```python
from build123d import *

# Parameters (mm, degrees)
F0_W      = 70
F0_H      = 52
F1_DEPTH  = 2.5
F2_R      = 0.5
F3_DEPTH  = 2
F5_DEPTH  = 7
F6_W      = 44
F6_H      = 52
F7_DEPTH  = 25
F10_W     = 48
F10_H     = 52
F11_DEPTH = 1.25
F12_W     = 48
F12_H     = 0.2
F12_H_2   = 0.75
F13_DEPTH = 0.375
F15_DEPTH = 60
F16_R     = 0.5
F17_DEPTH = 9
F18_R     = 0.5
F19_DEPTH = 9


# Not quite as in the source:
# - a feature names something its author has since deleted; it is built from what else it names


with BuildPart() as f1:
    # F0 (on Top) → F1 (new body)
    with BuildSketch(Plane.XY):
        with Locations((35, 26)):
            Rectangle(F0_W, F0_H)
    extrude(amount=F1_DEPTH)

    # F2 (on face) → F3 (cut)
    with BuildSketch(Plane(origin=(0, 0, 0), x_dir=(0, -1, 0), z_dir=(-1, 0, 0))):
        with Locations((-46, 1.25)):
            Circle(F2_R)
        with Locations((-38, 1.25)):
            Circle(F2_R)
        with Locations((-30, 1.25)):
            Circle(F2_R)
        with Locations((-22, 1.25)):
            Circle(F2_R)
        with Locations((-14, 1.25)):
            Circle(F2_R)
        with Locations((-6, 1.25)):
            Circle(F2_R)
    extrude(amount=-F3_DEPTH, mode=Mode.SUBTRACT)

    # F4 (on face) → F5 (join)
    with BuildSketch(Plane(origin=(0, 0, 0), x_dir=(0, -1, 0), z_dir=(-1, 0, 0))):
        with BuildLine():
            Line((-44.75, 0), (-44.75, 1.25))
            ThreePointArc((-44.75, 1.25), (-46, 2.5), (-47.25, 1.25))
            Line((-47.25, 1.25), (-47.25, 0))
            Line((-47.25, 0), (-44.75, 0))
        make_face()
        with BuildLine():
            Line((-36.75, 0), (-36.75, 1.25))
            ThreePointArc((-36.75, 1.25), (-38, 2.5), (-39.25, 1.25))
            Line((-39.25, 1.25), (-39.25, 0))
            Line((-39.25, 0), (-36.75, 0))
        make_face()
        with BuildLine():
            Line((-28.75, 0), (-28.75, 1.25))
            ThreePointArc((-28.75, 1.25), (-30, 2.5), (-31.25, 1.25))
            Line((-31.25, 1.25), (-31.25, 0))
            Line((-31.25, 0), (-28.75, 0))
        make_face()
        with BuildLine():
            Line((-20.75, 0), (-20.75, 1.25))
            ThreePointArc((-20.75, 1.25), (-22, 2.5), (-23.25, 1.25))
            Line((-23.25, 1.25), (-23.25, 0))
            Line((-23.25, 0), (-20.75, 0))
        make_face()
        with BuildLine():
            Line((-12.75, 0), (-12.75, 1.25))
            ThreePointArc((-12.75, 1.25), (-14, 2.5), (-15.25, 1.25))
            Line((-15.25, 1.25), (-15.25, 0))
            Line((-15.25, 0), (-12.75, 0))
        make_face()
        with BuildLine():
            Line((-4.75, 0), (-4.75, 1.25))
            ThreePointArc((-4.75, 1.25), (-6, 2.5), (-7.25, 1.25))
            Line((-7.25, 1.25), (-7.25, 0))
            Line((-7.25, 0), (-4.75, 0))
        make_face()
    extrude(amount=F5_DEPTH)

    # F6 (on face) → F7 (cut)
    with BuildSketch(Plane.XY.offset(2.5)):
        with Locations((48, 26)):
            Rectangle(F6_W, F6_H)
    extrude(amount=-F7_DEPTH, mode=Mode.SUBTRACT)

    # F9: F1 across plane


with BuildPart() as f1_1:
    add(f1.part)
    add(f1.part.mirror(Plane(origin=(26, 26, 1.25), x_dir=(0, 1, 0), z_dir=(1, 0, 0))))

    # F10 (on face) → F11 (cut)
    with BuildSketch(Plane.XY.offset(2.5)):
        with Locations((26, 26)):
            Rectangle(F10_W, F10_H)
    extrude(amount=-F11_DEPTH, mode=Mode.SUBTRACT)

    # F12 (on face) → F13 (cut)
    with BuildSketch(Plane.XY.offset(1.25)):
        with Locations((26, 6)):
            Rectangle(F12_W, F12_H)
        with Locations((26, 46)):
            Rectangle(F12_W, F12_H_2)
        Polygon((2, 14.15), (2, 14), (2, 13.85), (50, 13.85), (50, 14.15), align=None)
        Polygon((2, 22.2), (2, 22), (2, 21.8), (50, 21.8), (50, 22.2), align=None)
        Polygon((2, 30.25), (2, 30), (2, 29.75), (50, 29.75), (50, 30.25), align=None)
        Polygon((2, 38.3), (2, 38), (2, 37.7), (50, 37.7), (50, 38.3), align=None)
    extrude(amount=-F13_DEPTH, mode=Mode.SUBTRACT)

    # F14 (on face) → F15 (cut)
    with BuildSketch(Plane(origin=(0, 0, 0), x_dir=(0, -1, 0), z_dir=(-1, 0, 0))):
        Polygon((-51, 2.5), (-52, 2.5), (-52, 1.5), align=None)
        Polygon((-52, 1), (-52, 0), (-51, 0), align=None)
        Polygon((-1, 0), (0, 0), (0, 1), align=None)
        Polygon((0, 1.5), (0, 2.5), (-1, 2.5), align=None)
    extrude(amount=-F15_DEPTH, mode=Mode.SUBTRACT)

    # F16 (on face) → F17 (cut)
    with BuildSketch(Plane(origin=(-7, 0, 0), x_dir=(0, -1, 0), z_dir=(-1, 0, 0))):
        with Locations((-46, 1.25)):
            Circle(F16_R)
        with Locations((-38, 1.25)):
            Circle(F16_R)
        with Locations((-30, 1.25)):
            Circle(F16_R)
        with Locations((-22, 1.25)):
            Circle(F16_R)
        with Locations((-14, 1.25)):
            Circle(F16_R)
        with Locations((-6, 1.25)):
            Circle(F16_R)
    extrude(amount=-F17_DEPTH, mode=Mode.SUBTRACT)

    # F18 (on face) → F19 (cut)
    with BuildSketch(Plane.YZ.offset(59)):
        with Locations((6, 1.25)):
            Circle(F18_R)
        with Locations((14, 1.25)):
            Circle(F18_R)
        with Locations((22, 1.25)):
            Circle(F18_R)
        with Locations((30, 1.25)):
            Circle(F18_R)
        with Locations((38, 1.25)):
            Circle(F18_R)
        with Locations((46, 1.25)):
            Circle(F18_R)
    extrude(amount=-F19_DEPTH, mode=Mode.SUBTRACT)


solid = f1_1.part
```
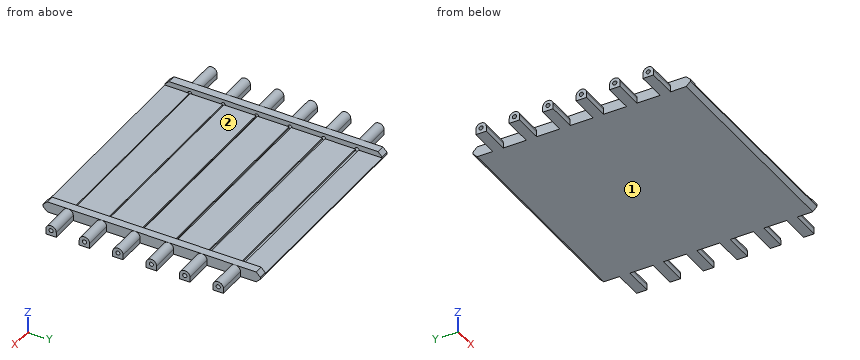
The model under review builds one solid part; all positions refer to its coordinate system, in mm. Face numbers are marked on the shaded views. Coordinates: 2 decimals unless noted, no trailing zeros. Write each loop counter-clockwise with the first axis right and the second up, starting at its lowest first coordinate (ties: lowest second). Pieces come first, ordered by that corner, then holes. Notation, with made-up numbers: (64, 29) -> (80, 29) arc R35 ccw to (80, 61) -> close; hole circle Ø9 at (83.5, 77.25). An arc over 180 degrees is marked (long way). One line per item, written item: value. Start each with the question number.
Q1. Clearance check with flat-ended pins moving along their axes: P1, Ø1, axis at x = 55.5, z = 1, coming from the +Y side; P2, Ø1.4, axis at x = 56, z = 1, coming from the -Y side; P3, Ø2.5, axis at x = 18, y = 26.5, coming from the +Z side. State where each tip first meets the part, or that it passes through.
Q2. The part is to be moulded in two halves that separate along X. For the marked faces 1 and 2, say which applies: +X half, -X half, draft (parallel to the pull), parting line (faces both ways), or undercut.
Q3. To check wall thickness, follow probe 1 along Y at (x, z) = (-3, 0.2); probe 2 along X at (y, z) = (26, 2.45); probe 3 along Z at (x, y) = (52, 6). State the ranges of each line that lie inside material, in increasing order.
Q4. Add section B-B, the plane y = 43. Give the boundary of the cut face in (x, z), then the cut area to 3 significant figures.
Response:
1. P1: y = 47.25
1. P2: y = 4.75
1. P3: z = 1.25
2. face 1: draft
2. face 2: undercut
3. probe 1: 4.75 to 7.25, 12.75 to 15.25, 20.75 to 23.25, 28.75 to 31.25, 36.75 to 39.25, 44.75 to 47.25
3. probe 2: 0 to 2, 50 to 52
3. probe 3: 0 to 0.75, 1.75 to 2.5
4. outline: (0, 0) -> (52, 0) -> (52, 2.5) -> (50, 2.5) -> (50, 1.25) -> (2, 1.25) -> (2, 2.5) -> (0, 2.5) -> close
4. area: 70.0 mm²
